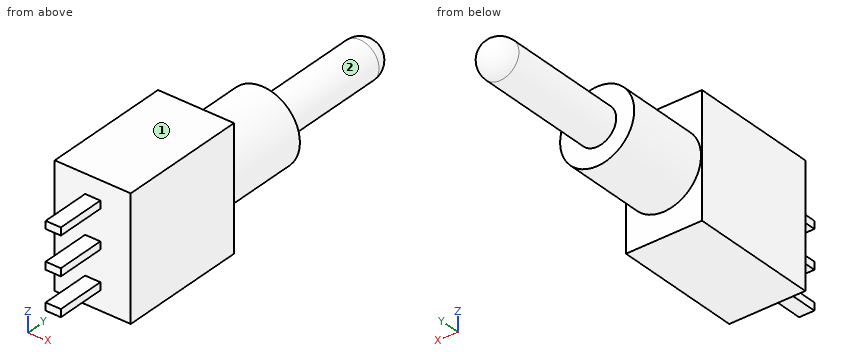
```python
from build123d import *

# Parameters (mm, degrees)
SKETCH1_W           = 5.08
SKETCH1_H           = 8.128
BOSS_EXTRUDE1_DEPTH = 8.636
SKETCH2_R           = 2.4765
BOSS_EXTRUDE2_DEPTH = 5.588
SKETCH3_W           = 1.016
SKETCH3_H           = 0.508
BOSS_EXTRUDE3_DEPTH = 3.302
SKETCH4_R           = 1.27
BOSS_EXTRUDE4_DEPTH = 9.398
FILLET1_R           = 1.27


with BuildPart() as part:
    # Sketch1 → Boss-Extrude1 (new body)
    with BuildSketch(Plane(origin=(0, 0, 0), x_dir=(1, 0, 0), z_dir=(0, 1, 0))):
        Rectangle(SKETCH1_W, SKETCH1_H)
    extrude(amount=BOSS_EXTRUDE1_DEPTH)

    # Sketch2 → Boss-Extrude2 (add)
    with BuildSketch(Plane(origin=(0, 8.636, 0), x_dir=(1, 0, 0), z_dir=(0, 1, 0))):
        with Locations(Location((0, 0, 0), (0, 0, 90))):
            Circle(SKETCH2_R)
    extrude(amount=BOSS_EXTRUDE2_DEPTH)

    # Sketch3 → Boss-Extrude3 (add)
    with BuildSketch(Plane.XZ):
        Rectangle(SKETCH3_W, SKETCH3_H)
        with Locations((0, -2.54)):
            Rectangle(SKETCH3_W, SKETCH3_H)
        with Locations((0, 2.54)):
            Rectangle(SKETCH3_W, SKETCH3_H)
    extrude(amount=BOSS_EXTRUDE3_DEPTH)

    # Sketch4 → Boss-Extrude4 (add)
    with BuildSketch(Plane(origin=(0, 14.224, 0), x_dir=(1, 0, 0), z_dir=(0, 1, 0))):
        with Locations(Location((0, 0, 0), (0, 0, 270))):
            Circle(SKETCH4_R)
    extrude(amount=BOSS_EXTRUDE4_DEPTH)

    # Fillet1
    fillet1_edges = [part.edges().sort_by_distance(p)[0] for p in [
        (0, 23.622, -1.27),
    ]]
    fillet(fillet1_edges, radius=FILLET1_R)


solid = part.part
```
Can you work these out from the model? Positions are in its coordinate system, mm. Face numbers are marked on the shaded views. A direction names the side the tool comes from. Give positions to 0.01 mm unless a question says otherwise; leave off trailing zeros. Order: outer loops, then holes, each group sorted by start corner. A loop starts at its lowest first (then second) coordinate and runs counter-clockwise, first axis right, second up. Notation, with made-up numbers: M -25,7 L 30,7 A21 cw 30,36 Z; hole C 2.25,61 d4. An arc over 180 degrees is marked long. One line per item, written item: value.
1) For P1, Ø0.6, axis at y = -1.5, z = -2.5, coming from the -X side; P2, Ø0.6, axis at y = -2, z = 2.5, coming from the +X side; P3, Ø0.5, axis at x = 0, y = -1, coming from the +Z side, each with a flat end and sliding along its axis, tell me the tip position at first contact or that it passes through.
Answer sheet:
P1: stops at x = -0.51
P2: stops at x = 0.51
P3: stops at z = 2.79
2) I want a section at C-C, the plane y = 13.75. List the corners of the cut face in (x, z) for me, plus the area to 3 significant figures.
Answer sheet:
outline: C 0,0 d4.95
area: 19.3 mm^2
3) On a 3-axis mill with a long thin cutter (end or side, diameter ignored), from which of +Z, -Z, +X, -X, +Y, -Y can I reach the whole of each face in a straight line? I mean the marked faces 1 and 2. Say none if no direction works.
Answer sheet:
face 1: +Z, +X, -X, +Y, -Y
face 2: +Y
4) I want a section at A-A, the plane x = 0. List the corners of the cut face in (y, z) for me, plus the area to 3 significant figures.
Answer sheet:
outline: M -3.3,-2.79 L 0,-2.79 L 0,-4.06 L 8.64,-4.06 L 8.64,-2.48 L 14.22,-2.48 L 14.22,-1.27 L 22.35,-1.27 A1.27 ccw 22.35,1.27 L 14.22,1.27 L 14.22,2.48 L 8.64,2.48 L 8.64,4.06 L 0,4.06 L 0,2.79 L -3.3,2.79 L -3.3,2.29 L 0,2.29 L 0,0.25 L -3.3,0.25 L -3.3,-0.25 L 0,-0.25 L 0,-2.29 L -3.3,-2.29 Z
area: 126 mm^2
5) I want a section at B-B, the plane z = 0. List the corners of the cut face in (x, y) for me, plus the area to 3 significant figures.
Answer sheet:
outline: M -2.54,0 L -0.51,0 L -0.51,-3.3 L 0.51,-3.3 L 0.51,0 L 2.54,0 L 2.54,8.64 L 2.48,8.64 L 2.48,14.22 L 1.27,14.22 L 1.27,22.35 A1.27 ccw -1.27,22.35 L -1.27,14.22 L -2.48,14.22 L -2.48,8.64 L -2.54,8.64 Z
area: 98.1 mm^2
6) Please list where these lines run through material, in increasing order: line 1 along Y through (x, z) = (0.1, -3.5); line 2 along Z through (x, y) = (-0.05, 13.75); line 3 along Y through (x, z) = (-1.9, 0.5).
Answer sheet:
line 1: y = 0 to 8.64
line 2: z = -2.48 to 2.48
line 3: y = 0 to 14.22
7) I want a section at D-D, the plane z = 1.75. List the corners of the cut face in (x, y) for me, plus the area to 3 significant figures.
Answer sheet:
outline: M -2.54,0 L 2.54,0 L 2.54,8.64 L 1.75,8.64 L 1.75,14.22 L -1.75,14.22 L -1.75,8.64 L -2.54,8.64 Z
area: 63.5 mm^2
